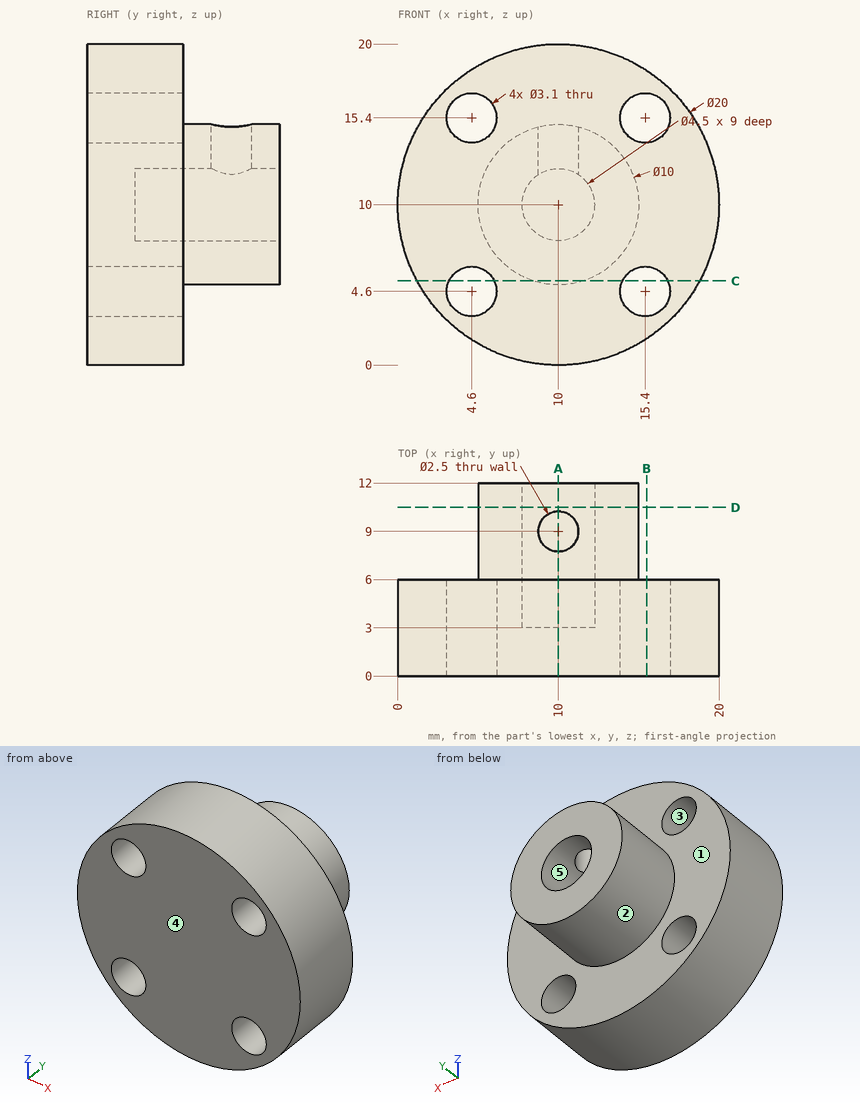
Answer from the drawing. Dimensions are ordinates in mm from the lowest x, y and z of the part. A direction names the side the tool comes from. Round coordinates to 2 decimals unless told otherwise and drop trailing zeros. Write each loop counter-clockwise with the first axis right and the second up, starting at its lowest first coordinate (ties: lowest second). Pieces come first, ordered by that corner, then holes. Notation, with made-up numbers: (57, 7.25) - (93, 7.25) arc R16 cw to (93, 35.25) - close; hole circle Ø10 at (66.25, 53.25). An arc over 180 degrees is marked (long way). Use a Markdown table: item, result.
(1) Each of these flat-tipped pins is pushed along its axis until it touches: pin 1 Ø1.5 at (x, y) = (10, 9) entering from -Z; pin 2 Ø4 at (y, z) = (10, 10) entering from +X; pin 3 Ø1.5 at (x, y) = (11, 2) entering from +Z. Where does it stop, or does it pass through?
Reported:
| item | result |
|---|---|
| pin 1 | z = 5 |
| pin 2 | x = 15 |
| pin 3 | z = 20 |
(2) The part is cut by section A-A (x = 10). Write down the section's boundary in (y, z), then the cut area to 3 significant figures.
Reported:
| item | result |
|---|---|
| outline | (0, 0) - (6, 0) - (6, 5) - (12, 5) - (12, 7.75) - (3, 7.75) - (3, 12.25) - (7.75, 12.25) - (7.75, 15) - (6, 15) - (6, 20) - (0, 20) - close; (10.25, 12.25) - (12, 12.25) - (12, 15) - (10.25, 15) - close |
| area | 133 mm2 |
(3) The part is cut by section B-B (x = 15.5). Write down the section's boundary in (y, z), then the cut area to 3 significant figures.
Reported:
| item | result |
|---|---|
| outline | (0, 1.65) - (6, 1.65) - (6, 3.05) - (0, 3.05) - close; (0, 6.15) - (6, 6.15) - (6, 13.85) - (0, 13.85) - close; (0, 16.95) - (6, 16.95) - (6, 18.35) - (0, 18.35) - close |
| area | 63.1 mm2 |
(4) The mould has two halves that part along Z. Classify the marked faces 1, 2 and 3: released by +Z, released by -Z, zero draft, split by the parting line, or undercut.
Reported:
| item | result |
|---|---|
| face 1 | zero draft |
| face 2 | split by the parting line |
| face 3 | undercut |
(5) Which of the six approach directions +Z, -Z, +X, -X, +Y, -Y give full straight-line access (tool end or side, diameter ignored) to the marked faces 4 and 5?
Reported:
| item | result |
|---|---|
| face 4 | +Z, -Z, +X, -X, -Y |
| face 5 | +Y |
(6) The part is cut by section C-C (z = 5.25). Write down the section's boundary in (x, y).
Reported:
| item | result |
|---|---|
| outline | (1.2, 0) - (3.19, 0) - (3.19, 6) - (1.2, 6) - close; (6.01, 0) - (13.99, 0) - (13.99, 6) - (11.56, 6) - (11.56, 12) - (8.44, 12) - (8.44, 6) - (6.01, 6) - close; (16.81, 0) - (18.8, 0) - (18.8, 6) - (16.81, 6) - close |
(7) The part is cut by section D-D (y = 10.5). Write down the section's boundary in (x, z), then the cut area to 3 significant figures.
Reported:
| item | result |
|---|---|
| outline | circle Ø10 at (10, 10); hole circle Ø4.5 at (10, 10) |
| area | 62.6 mm2 |
(8) Straight lines are drawn through the part: line 1 along Z through (x, y) = (15.4, 4.7); line 2 along Y through (x, z) = (10, 13.05); line 3 along X through (y, z) = (10.25, 10). For each, find the intervals that lie inside material, in ascending order. Write a range as [from, to].
Reported:
| item | result |
|---|---|
| line 1 | [1.58, 3.05], [6.15, 13.85], [16.95, 18.42] |
| line 2 | [0, 7.75], [10.25, 12] |
| line 3 | [5, 7.75], [12.25, 15] |
